```python
from build123d import *

# Parameters (mm, degrees)
F1_DEPTH = 5
F2_W     = 4
F2_H     = 4
F4_W     = 4
F4_H     = 4
F7_W     = 2
F7_H     = 3
F9_W     = 2
F9_H     = 5
F11_W    = 3
F11_H    = 30
F13_W    = 3
F13_H    = 31
F16_R    = 5


with BuildPart() as f1:
    # F0 (on Top) → F1 (new body)
    with BuildSketch(Plane.XY):
        with BuildLine():
            Line((-30, 0), (0, 0))
            Line((0, 0), (0, 25))
            Line((0, 25), (-25, 25))
            ThreePointArc((-25, 25), (-28.5355339059, 23.5355339059), (-30, 20))
            Line((-30, 20), (-30, 0))
        make_face()
    extrude(amount=F1_DEPTH)

    # F2 (on face) → F5 section 0
    with BuildSketch(Plane(origin=(0, 0, 0), x_dir=(1, 0, 0), z_dir=(0, 0, -1))):
        with Locations((-24, -19)):
            Rectangle(F2_W, F2_H)
    # F4 (on offset) → F5 section 1
    with BuildSketch(Plane(origin=(0, 0, -35), x_dir=(1, 0, 0), z_dir=(0, 0, -1))):
        with Locations((-27, -22)):
            Rectangle(F4_W, F4_H)
    loft()

    # F6: F1 across plane


with BuildPart() as f1_1:
    add(f1.part)
    add(f1.part.mirror(Plane.YZ))

    # F7 (on face) → F10 section 0
    with BuildSketch(Plane.XY.offset(5)):
        with Locations((24.9823927879, 19)):
            Rectangle(F7_W, F7_H)
    # F9 (on offset) → F10 section 1
    with BuildSketch(Plane.XY.offset(30)):
        with Locations((28.6593784243, 25.6122151948)):
            Rectangle(F9_W, F9_H)
    loft()

    # F11 (on offset) → F14 section 0
    with BuildSketch(Plane.XY.offset(30)):
        with Locations((28.6593784243, 15)):
            Rectangle(F11_W, F11_H)
    # F13 (on offset) → F14 section 1
    with BuildSketch(Plane.XY.offset(60)):
        with Locations((29.6593784243, 15.5)):
            Rectangle(F13_W, F13_H)
    loft()

    # F15: F1 across plane


with BuildPart() as f1_2:
    add(f1_1.part)
    add(f1_1.part.mirror(Plane.XZ))

    # F16
    f16_edges = [f1_2.edges().sort_by_distance(p)[0] for p in [
        (29.659378, 31, 60),
        (29.659378, -31, 60),
    ]]
    fillet(f16_edges, radius=F16_R)

    # F17: F1 across plane


with BuildPart() as f1_3:
    add(f1_2.part)
    add(f1_2.part.mirror(Plane.XZ))


solid = f1_3.part
```
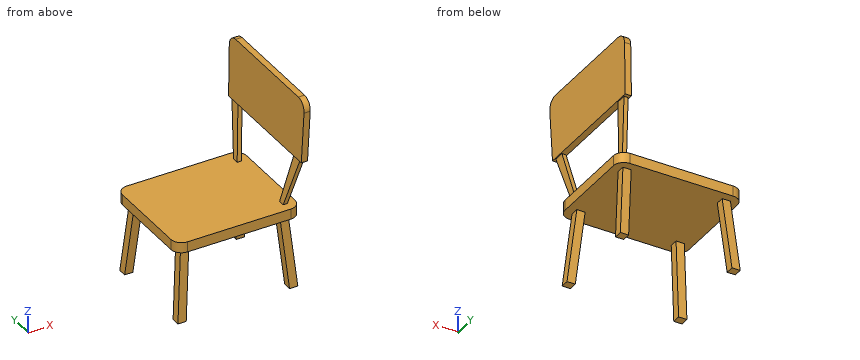
Read the model definition and answer for the solid it produces. Units are mm, in the model's axes. Give positions to 0.01 mm unless a question says otherwise; leave off trailing zeros. Write each loop counter-clockwise with the first axis right and the second up, starting at its lowest first coordinate (ties: lowest second). Pieces come first, ordered by that corner, then holes. Notation, with made-up numbers: (-25.5, 71.25) -> (-0.5, 71.25) arc R30 cw to (-0.5, 108.25) -> close; hole circle Ø8 at (57, -26). An arc over 180 degrees is marked (long way). Answer as a JSON object with one key per item and string values.
1) Flat-ended cylindrical pins translate along their axes: pin 1 Ø10 at (y, z) = (17.5, 48) entering from +X; pin 2 Ø1.5 at (x, z) = (-4.5, 2) entering from -Y; pin 3 Ø6 at (x, y) = (-6.5, 5.5) entering from -Z. Find the tip coordinate at first contact, or state that the pin passes through.
Findings below:
{"pin 1": "stops at x = 30.93", "pin 2": "stops at y = -25", "pin 3": "stops at z = 0"}
2) Section A-A on y = 1 is taken. Write down the section's boundary in (x, z).
Findings below:
{"outline": "(-30, 0) -> (30, 0) -> (30, 5) -> (-30, 5) -> close; (27.16, 30) -> (30.16, 30) -> (31.16, 60) -> (28.16, 60) -> close"}
3) Section C-C on z = -2.5 is taken. Count the separate pieces of the cut face and the enclosed holes in it, then the cut area to 3 significant figures.
Findings below:
{"separate pieces": "4", "enclosed holes": "0", "area": "64.0 mm^2"}
4) Section B-B on x = 4 is taken. Write down the section's boundary in (y, z).
Findings below:
{"outline": "(-25, 0) -> (25, 0) -> (25, 5) -> (-25, 5) -> close"}
5) Straight lines are drawn through the part: probe 1 along Z at (x, y) = (-5, -2); probe 2 along Y at (x, z) = (27, -24); probe 3 along X at (y, z) = (-22.5, -28). For each, find the intervals that lie inside material, in ascending order. Write a range as from..to.
Findings below:
{"probe 1": "z = 0..5", "probe 2": "y = -23.06..-19.06, 19.06..23.06", "probe 3": "x = -28.4..-24.4, 24.4..28.4"}
